from build123d import *

# Parameters (mm, degrees)
BOSS_EXTRUDE1_DEPTH = 5
SKETCH2_R           = 0.5
CUT_EXTRUDE1_DEPTH  = 9.660254038
BOSS_EXTRUDE2_DEPTH = 2.5


with BuildPart() as part:
    # Sketch1 → Boss-Extrude1 (new body)
    with BuildSketch(Plane.XY):
        with BuildLine():
            Line((0, 5), (2.5, 5))
            ThreePointArc((2.5, 5), (5, 2.5), (2.5, 0))
            Line((2.5, 0), (0, 0))
            Line((0, 0), (0, 5))
        make_face()
    extrude(amount=BOSS_EXTRUDE1_DEPTH)

    # Sketch2 → Cut-Extrude1 (cut, through all)
    with BuildSketch(Plane.XY):
        with Locations((2.5, 2.5)):
            Circle(SKETCH2_R)
    extrude(amount=CUT_EXTRUDE1_DEPTH, mode=Mode.SUBTRACT)

    # Sketch4 → Boss-Extrude2 (add)
    with BuildSketch(Plane.ZY):
        Polygon((2.25, 2.75), (2.25, 3.25), (2.75, 3.25), (2.75, 2.75), (3.75, 2.75), (3.75, 2.25), (2.75, 2.25), (2.75, 1.75), (2.25, 1.75), (2.25, 2.25), (1.25, 2.25), (1.25, 2.75), align=None)
    extrude(amount=BOSS_EXTRUDE2_DEPTH)


solid = part.part
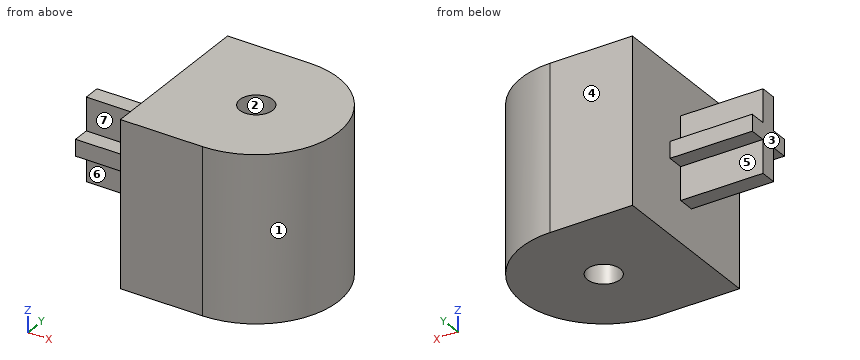
Geometry check sheet. Reference: the model listing, model coordinates, mm. Face numbers are marked on the shaded views. A direction names the side the tool comes from. Give positions to 0.01 mm unless a question says otherwise; leave off trailing zeros. Loops run counter-clockwise (first coordinate to the right, second up) from the corner with the lowest first, then second, coordinate; pieces in that order, holes last. Notation, with made-up numbers: M -32.5,11 L -16.5,11 A17 ccw -16.5,18 Z; hole C 50,16.5 d1. An arc over 180 degrees is marked long. Answer as a JSON object with one key per item and string values. Group by question number.
Item 1: Access from +Z, -Z, +X, -X, +Y, -Y to the whole of each face (thin tool, end or side, straight path). Record for the marked faces 5, 6 and 7.
Item 2: Sectioned sample at D-D on y = 0.5. Record the boundary of the cut face in (x, z), plus the area to 3 significant figures.
Item 3: Sectioned sample at C-C on x = -1.5. Record the boundary of the cut face in (y, z), plus the area to 3 significant figures.
Item 4: Sectioned sample at A-A on y = 2.5. Record the boundary of the cut face in (x, z).
Item 5: Gauge pin test, flat ends, axial feed: pin 1 (0.8 mm diameter, centred on x = -1, z = 3.5, fed in from -Y); pin 2 (0.5 mm diameter, centred on x = -1.5, z = 3.5, fed in from +Y); pin 3 (1.1 mm diameter, centred on x = -2, z = 2, fed in from +Y). Record the tip position at first contact, or that the pin passes through.
Item 6: Sectioned sample at B-B on z = 4.25. Record the boundary of the cut face in (x, y), plus the area to 3 significant figures.
Item 7: Mould release check, pull along X, two halves, no side actions. Record for the marked faces 1, 2, 3 and 4: pulls with the +X half, pulls with the -X half, needs draft (parallel to the pull), parting line crosses it, or undercut.
Item 8: Material ranges on L1, parallel to X at y = 2.5, z = 2.9; L2, parallel to Y at x = 2.5, z = 1.5; L3, parallel to Y at x = -2, z = 1.75, recorded low to high.
Findings below:
{
 "1": {"face 5": "-Z, -X, +Y", "face 6": "-Z, -X, -Y", "face 7": "+Z, -X, -Y"},
 "2": {"outline": "M 0,0 L 4,0 L 4,5 L 0,5 Z", "area": "20.0 mm2"},
 "3": {"outline": "M 1.75,2.25 L 2.25,2.25 L 2.25,1.25 L 2.75,1.25 L 2.75,2.25 L 3.25,2.25 L 3.25,2.75 L 2.75,2.75 L 2.75,3.75 L 2.25,3.75 L 2.25,2.75 L 1.75,2.75 Z", "area": "1.75 mm2"},
 "4": {"outline": "M -2.5,1.25 L 0,1.25 L 0,0 L 2,0 L 2,5 L 0,5 L 0,3.75 L -2.5,3.75 Z; M 3,0 L 5,0 L 5,5 L 3,5 Z"},
 "5": {"pin 1": "y = 2.25", "pin 2": "y = 2.75", "pin 3": "y = 3.25"},
 "6": {"outline": "M 0,0 L 2.5,0 A2.5 ccw 2.5,5 L 0,5 Z; hole C 2.5,2.5 d1", "area": "21.5 mm2"},
 "7": {"face 1": "pulls with the +X half", "face 2": "undercut", "face 3": "pulls with the -X half", "face 4": "needs draft"},
 "8": {"L1": "-2.5 to 2, 3 to 5", "L2": "0 to 2, 3 to 5", "L3": "2.25 to 2.75"}
}
